Verification items for this drawing (mm, ordinates from the low corner). Coordinates: 2 decimals unless noted, no trailing zeros. Loops run counter-clockwise (first coordinate to the right, second up) from the corner with the lowest first, then second, coordinate; pieces in that order, holes last. Notation, with made-up numbers: M 29,59 L 59,59 A24 ccw 59,75 Z; hole C -5.75,-5.5 d6. An arc over 180 degrees is marked long. Use CSV: the item, a comma, the result in double quotes.
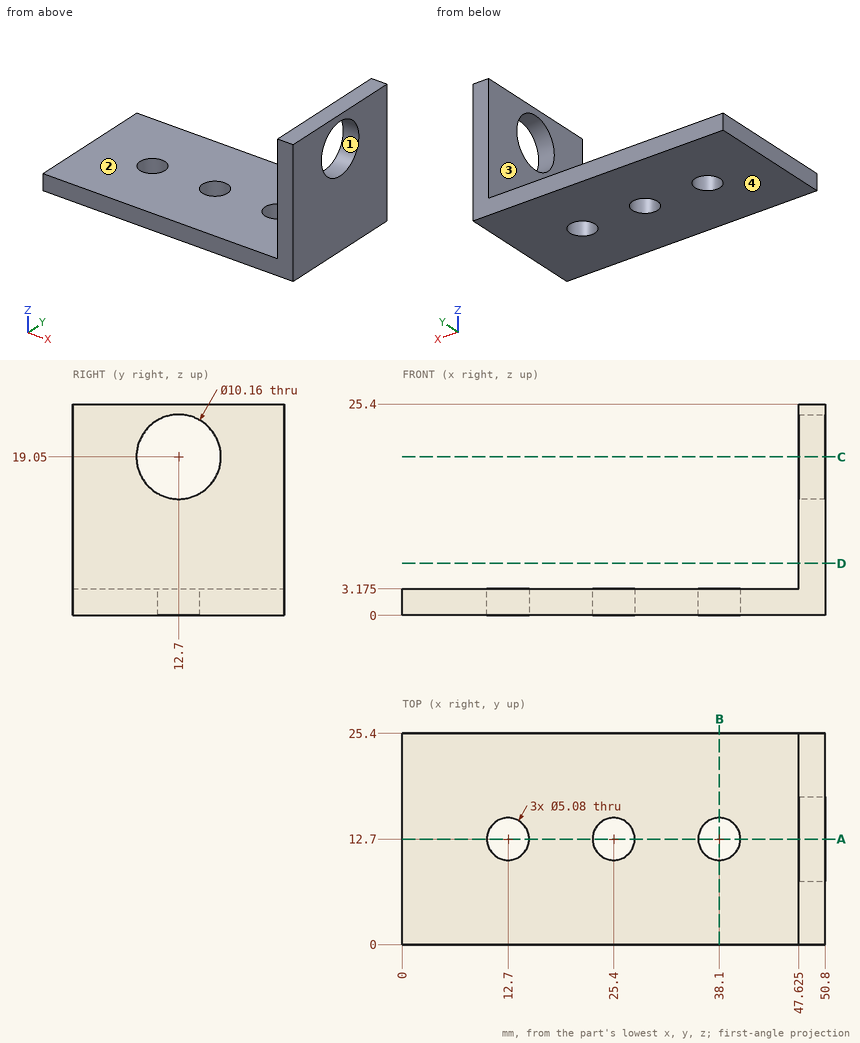
1. Section check D-D, the plane z = 6.25. Record the cut outline in (x, y) (3 decimals).
The answers:
outline,"M 47.625,0 L 50.8,0 L 50.8,25.4 L 47.625,25.4 Z"
2. Section check B-B, the plane x = 38.1. Record the cut outline in (y, z) (3 decimals), plus the area to 3 significant figures.
The answers:
outline,"M 0,0 L 10.16,0 L 10.16,3.175 L 0,3.175 Z; M 15.24,0 L 25.4,0 L 25.4,3.175 L 15.24,3.175 Z"
area,"64.5 mm^2"
3. Section check A-A, the plane y = 12.7. Record the cut outline in (x, z) (3 decimals).
The answers:
outline,"M 0,0 L 10.16,0 L 10.16,3.175 L 0,3.175 Z; M 15.24,0 L 22.86,0 L 22.86,3.175 L 15.24,3.175 Z; M 27.94,0 L 35.56,0 L 35.56,3.175 L 27.94,3.175 Z; M 40.64,0 L 50.8,0 L 50.8,13.97 L 47.625,13.97 L 47.625,3.175 L 40.64,3.175 Z; M 47.625,24.13 L 50.8,24.13 L 50.8,25.4 L 47.625,25.4 Z"
4. Thickness scan on line 1 (Y direction, x = 25.4, z = 2.3); line 2 (Y direction, x = 48.6, z = 19.05); line 3 (Z direction, x = 43.5, y = 5.75) (3 decimals). Record the ranges inside material, lowest first. Write a range as [from, to].
The answers:
line 1,"[0, 10.16], [15.24, 25.4]"
line 2,"[0, 7.62], [17.78, 25.4]"
line 3,"[0, 3.175]"
5. Release check for a two-part mould opening along Z. For the marked faces 1, 2, 3 and 4 record: +Z half, -Z half, draft (parallel to the pull), parting line (faces both ways), or undercut.
The answers:
face 1,"undercut"
face 2,"+Z half"
face 3,"draft"
face 4,"-Z half"
6. Gauge pin test, flat end, axial feed: P1, Ø8, axis at x = 12.7, y = 12.7, coming from the +Z side (3 decimals). Record the tip position at first contact, or that the pin passes through.
The answers:
P1,"z = 3.175"
7. Section check C-C, the plane z = 19.05. Record the cut outline in (x, y) (3 decimals), plus the area to 3 significant figures.
The answers:
outline,"M 47.625,0 L 50.8,0 L 50.8,7.62 L 47.625,7.62 Z; M 47.625,17.78 L 50.8,17.78 L 50.8,25.4 L 47.625,25.4 Z"
area,"48.4 mm^2"
